Build history of the part. All positions in model axes, mm. Give positions to 0.01 mm unless a question says otherwise; leave off trailing zeros. Write each loop counter-clockwise with the first axis right and the second up, starting at its lowest first coordinate (ties: lowest second). Pieces come first, ordered by that corner, then holes. Notation, with made-up numbers: M -6.75,19.5 L 23.25,19.5 A9 ccw 23.25,27.5 Z; hole C 18,-36 d5. An arc over 180 degrees is marked long. One line per item, written item: value. Start each with the question number.
from build123d import *

# Parameters (mm, degrees)
F1_DEPTH = 97.6482406259


# Not quite as in the source:
# - the program builds the solid bodies; features that only make, move or delete a surface that nothing else refers to are left out


with BuildPart() as f1:
    # F0 (on Front) → F1 (new body)
    with BuildSketch(Plane.XZ):
        Polygon((47.9935407639, 0), (-47.9935407639, 0), (-47.9935407639, -55.3510189056), (48.1260120869, -55.3510189056), (48.1260120869, 0), align=None)
        with BuildLine():
            ThreePointArc((47.9935407639, 0), (0, 47.9935407639), (-47.9935407639, 0))
            Line((-47.9935407639, 0), (47.9935407639, 0))
        make_face()
    extrude(amount=F1_DEPTH)


solid = f1.part
1) Drop flat-ended pins along their axis: P1, Ø1, axis at x = -20, y = -39.5, coming from the +Z side; P2, Ø6, axis at x = 6.5, y = -24, coming from the +Z side; P3, Ø1.5, axis at x = 24, y = -28.5, coming from the +Z side. Give the stop position or say it passes through.
2) Probe line 1 along Z through (x, y) = (1, -12); line 2 along Z through (x, y) = (21.5, -31.5); line 3 along X through (y, z) = (-44, 15). List the from-to ranges inside material, lowest first. Write a range as from..to.
3) Band-saw the part on C-C (z = 22). List the corners of the cut face in (x, y), then the cut area to 3 significant figures.
4) Band-saw the part on A-A (y = -81.5). List the corners of the cut face in (x, z), then the cut area to 3 significant figures.
5) Band-saw the part on B-B (x = -13). List the corners of the cut face in (y, z).
Model answer:
1. P1: stops at z = 43.85
1. P2: stops at z = 47.87
1. P3: stops at z = 41.99
2. line 1: z = -55.35..47.98
2. line 2: z = -55.35..42.91
2. line 3: x = -45.59..45.59
3. outline: M -42.65,-97.65 L 42.65,-97.65 L 42.65,0 L -42.65,0 Z
3. area: 8,330 mm²
4. outline: M -47.99,-55.35 L 48.13,-55.35 L 48.13,0 L 47.99,0 A47.99 ccw -47.99,0 Z
4. area: 8,940 mm²
5. outline: M -97.65,-55.35 L 0,-55.35 L 0,46.2 L -97.65,46.2 Z
